For this review, take the finished solid that the model builds, in its own axes (mm). Round coordinates to 2 decimals unless told otherwise and drop trailing zeros. Write each loop counter-clockwise with the first axis right and the second up, starting at its lowest first coordinate (ties: lowest second). Pieces come first, ordered by that corner, then holes. Notation, with made-up numbers: M 75.25,73 L 120.25,73 A12 ccw 120.25,80 Z; hole C -13,77.5 d5. An arc over 180 degrees is marked long. Use one line per item in the form item = value. Start each with the question number.
Item 1: For line 1 (Y direction, x = 12.7, z = 33.5) (3 decimals); line 2 (Y direction, x = 7, z = 50.5); line 3 (X direction, y = -5, z = 6), list the stretches that pass through material, from the lowest coordinate up. Write a range as [from, to].
Item 2: For P1, Ø10, axis at x = 12.7, y = -9.525, coming from the +Z side, flat-tipped, find the tip position at first contact; note if it passes through.
Item 3: Add section A-A (x = 12.7). State the section outline as (y, z) points (3 decimals).
Item 4: Add section B-B (y = -10.5). State the section outline as (x, z) points, and give its area (3 significant figures).
Item 5: Add section C-C (z = 53). State the section outline as (x, y) points (3 decimals).
Item 6: Draft analysis for pull direction X (two halves, no side actions). For faces 1 (the cylindrical face through (8.02, -5.233, 38.633)), 2 (the cylindrical face through (-23.951, -5.994, 74.672)), 3 (the flat face through (38.1, -7, 35)), state which applies: released by +X, released by -X, zero draft, split by the parting line, or undercut.
from build123d import *

# Parameters (mm, degrees)
F0_W     = 63.5
F0_H     = 50.8
F1_DEPTH = 76.2
F2_R     = 6.35
F3_DEPTH = 76.201
F4_SIZE  = 5.08
F5_R     = 5.08


with BuildPart() as f1:
    # F0 (on Top) → F1 (new body)
    with BuildSketch(Plane.XY):
        with Locations((6.35, -6.35)):
            Rectangle(F0_W, F0_H)
    extrude(amount=F1_DEPTH)

    # F2 (on face) → F3 (cut, through all)
    with BuildSketch(Plane.XY.offset(76.2)):
        with Locations((12.7, -9.525)):
            Circle(F2_R)
    extrude(amount=-F3_DEPTH, mode=Mode.SUBTRACT)

    # F4
    f4_edges = [f1.edges().sort_by_distance(p)[0] for p in [
        (6.35, 19.05, 76.2),
        (6.35, -31.75, 76.2),
    ]]
    chamfer(f4_edges, length=F4_SIZE)

    # F5
    f5_edges = [f1.edges().sort_by_distance(p)[0] for p in [
        (-25.4, -6.35, 76.2),
        (38.1, -6.35, 76.2),
    ]]
    fillet(f5_edges, radius=F5_R)


solid = f1.part
Calculated:
q1.line_1 = [-31.75, -15.875], [-3.175, 19.05]
q1.line_2 = [-31.75, -12.32], [-6.73, 19.05]
q1.line_3 = [-25.4, 8.25], [17.15, 38.1]
q2.P1 = through
q3.outline = M -31.75,0 L -15.875,0 L -15.875,76.2 L -26.67,76.2 L -31.75,71.12 Z; M -3.175,0 L 19.05,0 L 19.05,71.12 L 13.97,76.2 L -3.175,76.2 Z
q4.outline = M -25.4,0 L 6.43,0 L 6.43,76.2 L -20.32,76.2 A5.08 ccw -25.4,71.12 Z; M 18.97,0 L 38.1,0 L 38.1,71.12 A5.08 ccw 33.02,76.2 L 18.97,76.2 Z
q4.area = 3,870 mm^2
q5.outline = M -25.4,-31.75 L 38.1,-31.75 L 38.1,19.05 L -25.4,19.05 Z; hole C 12.7,-9.525 d12.7
q6.face_1 = undercut
q6.face_2 = released by -X
q6.face_3 = released by +X
